Source: three-view drawing plus pictorial views. Frame: mm from the lowest corner of the part. A direction names the side the tool comes from. Give positions to 0.01 mm unless a question says otherwise; leave off trailing zeros. Order: outer loops, then holes, each group sorted by start corner. A loop starts at its lowest first (then second) coordinate and runs counter-clockwise, first axis right, second up. Notation, with made-up numbers: (48.5, -16.75) -> (52.5, -16.75) arc R32 ccw to (52.5, 13.25) -> close; hole circle Ø4 at (36.5, -3.5). An arc over 180 degrees is marked (long way). Use a Markdown table: item, result. Add a question column.
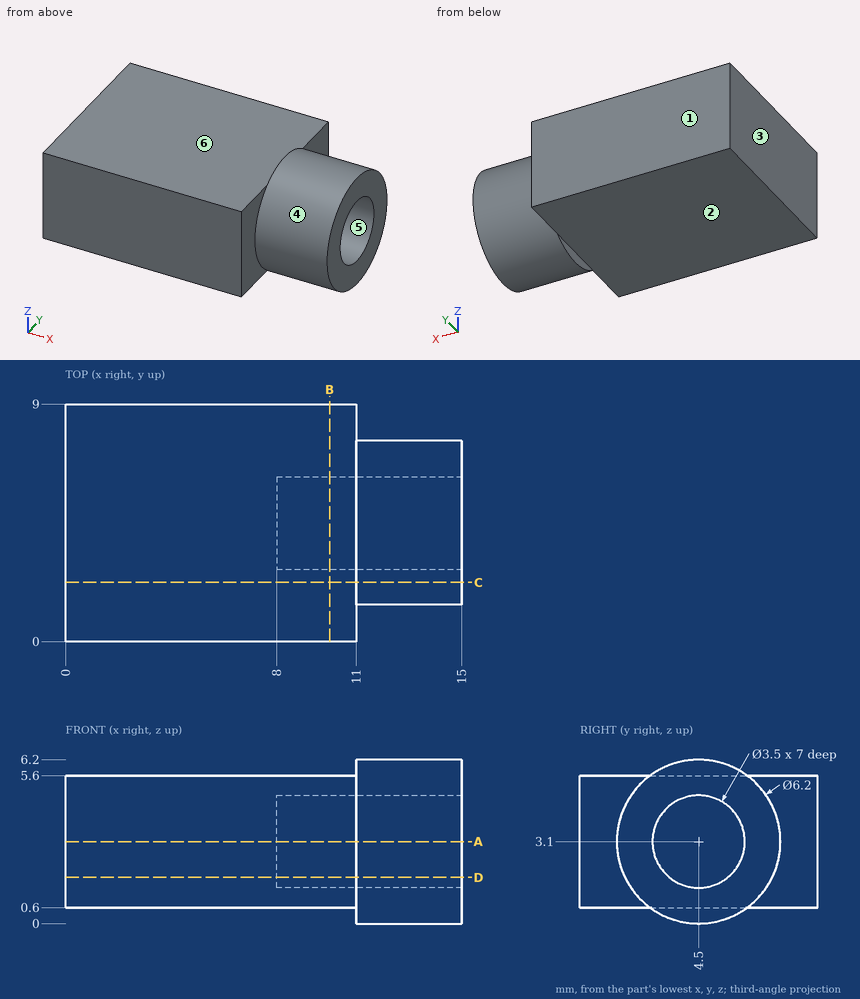
Q1. Section query A-A (z = 3.1). Return loops of the section in (x, y), plus the area to 3 significant figures.
Q2. Section query B-B (x = 10). Return loops of the section in (y, z), plus the area to 3 significant figures.
Q3. Draft query along Z for the marked faces 3, 4, 5 and 6. Return one class per face: +Z half, -Z half, draft (parallel to the pull), parting line (faces both ways), or undercut.
Q4. Section query C-C (y = 2.25). Return loops of the section in (x, z).
Q5. Section query D-D (z = 1.75). Return loops of the section in (x, y).
Q6. First-contact query: pin 1 (0.7 mm diameter, centred on y = 4.5, z = 0, fed in from -X); pin 2 (2 mm diameter, centred on y = 4.5, z = 3.1, fed in from +X); pin 3 (1.5 mm diameter, centred on x = 10, y = 4.5, fed in from -Z). Flat tips, straight axial feed; report the tip coordinate or a pass-through.
Q7. Access query for the marked faces 1 and 2. Directions: +Z, -Z, +X, -X, +Y, -Y. A direction counts if a zero-diameter tool reaches every point of the face in a straight line with its end or side. Return the directions, or none.
Q8. Ray query, line 1 (Y direction, x = 13, z = 3); line 2 (Z direction, x = 2.75, y = 0.75); line 3 (X direction, y = 8.5, z = 4.5). Return the intervals inside material, ascending.
Solution:
| question | item | result |
|---|---|---|
| 1 | outline | (0, 0) -> (11, 0) -> (11, 1.4) -> (15, 1.4) -> (15, 2.75) -> (8, 2.75) -> (8, 6.25) -> (15, 6.25) -> (15, 7.6) -> (11, 7.6) -> (11, 9) -> (0, 9) -> close |
| 1 | area | 99.3 mm² |
| 2 | outline | (0, 0.6) -> (9, 0.6) -> (9, 5.6) -> (0, 5.6) -> close; hole circle Ø3.5 at (4.5, 3.1) |
| 2 | area | 35.4 mm² |
| 3 | face 3 | draft |
| 3 | face 4 | parting line |
| 3 | face 5 | undercut |
| 3 | face 6 | +Z half |
| 4 | outline | (0, 0.6) -> (11, 0.6) -> (11, 0.97) -> (15, 0.97) -> (15, 5.23) -> (11, 5.23) -> (11, 5.6) -> (0, 5.6) -> close |
| 5 | outline | (0, 0) -> (11, 0) -> (11, 1.71) -> (15, 1.71) -> (15, 3.39) -> (8, 3.39) -> (8, 5.61) -> (15, 5.61) -> (15, 7.29) -> (11, 7.29) -> (11, 9) -> (0, 9) -> close |
| 6 | pin 1 | stops at x = 11 |
| 6 | pin 2 | stops at x = 8 |
| 6 | pin 3 | stops at z = 0.6 |
| 7 | face 1 | +Z, -Z, +X, -X, +Y |
| 7 | face 2 | -Z, -X, +Y, -Y |
| 8 | line 1 | y = 1.4 to 2.75, 6.25 to 7.6 |
| 8 | line 2 | z = 0.6 to 5.6 |
| 8 | line 3 | x = 0 to 11 |
